from build123d import *

# Parameters (mm, degrees)
F0_R     = 53.0991394176
F1_DEPTH = 51.71754
F0_R_2   = 55.7255834594
F2_DEPTH = 232.41034
F3_T     = -2.54
F4_DEPTH = 228.21454
F5_T     = -2.54


# Not quite as in the source:
# - a shell that OpenCascade refuses in one call is made with other operations: the cavity is built on its own and cut out


with BuildPart() as f1:
    # F0 (on Top) → F1 (new body)
    with BuildSketch(Plane.XY):
        Circle(F0_R)
    extrude(amount=F1_DEPTH)

    # F3
    f3_openings = [f1.faces().sort_by_distance(p)[0] for p in [
        (0, 0, 51.71754),
    ]]
    offset(amount=F3_T, openings=f3_openings)

    # F4 (add): a face of the model
    f4_faces = [f1.faces().sort_by_distance(p)[0] for p in [
        (0, 0, 0),
    ]]


with BuildPart() as f2:
    # F0 (on Top) → F2 (new body)
    with BuildSketch(Plane.XY):
        Circle(F0_R_2)
        Circle(F0_R, mode=Mode.SUBTRACT)
    extrude(amount=-F2_DEPTH)


with BuildPart() as f1_1:
    add(f1.part)

    add(f2.part)  # F4 merges F2
    extrude(f4_faces, amount=F4_DEPTH)

    # F5: a shell. OpenCascade refuses it in one call, so the cavity is built on its own and cut out:
    # the body offset inwards by the wall thickness, plus a prism from it out through each open face.
    f5_core = offset(f1_1.part, amount=F5_T, kind=Kind.INTERSECTION, mode=Mode.PRIVATE)
    f5_exits = [f5_core.faces().sort_by_distance(p)[0] for p in [
        (0, 0, 0),
    ]]
    add(f5_core, mode=Mode.SUBTRACT)
    extrude(f5_exits, amount=-F5_T, mode=Mode.SUBTRACT)


solid = f1_1.part
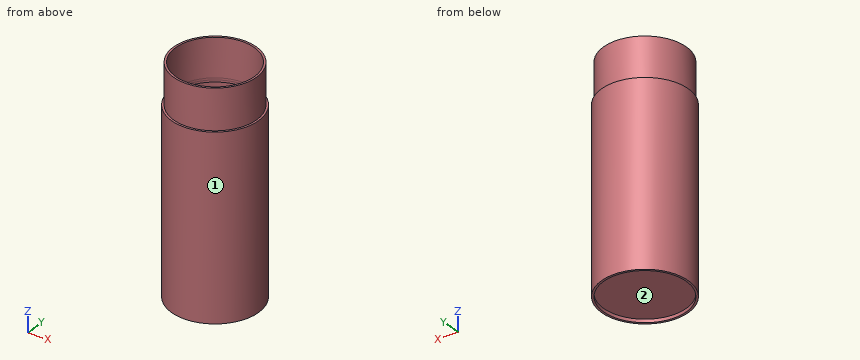
Source: CAD feature listing. Evaluate the final solid. Frame: model axes, mm. Face numbers are marked on the shaded views. Coordinates: 2 decimals unless noted, no trailing zeros. Order: outer loops, then holes, each group sorted by start corner. A loop starts at its lowest first (then second) coordinate and runs counter-clockwise, first axis right, second up. Notation, with made-up numbers: M 77.5,28.25 L 130.5,28.25 A21 cw 130.5,45.25 Z; hole C -2,60 d1. An arc over 180 degrees is marked long. Write each question's results on one line, items separated by ' | '. Start each with the question number.
1. Section D-D, the plane z = 21. Return the cut outline in (x, y).
2. Draft query along Y for the marked faces 1 and 2. Return one class per face: +Y half, -Y half, draft (parallel to the pull), parting line (faces both ways), or undercut.
3. Section C-C, the plane z = -89.5. Return the cut outline in (x, y), then the cut area to 3 significant figures.
4. Material intervals for L1, parallel to Z at x = 3, y = 51.5; L2, parallel to Y at x = 0, z = 33; L3, parallel to Y at x = 2, z = -15, sorted ascending.
5. Section A-A, the plane y = 0. Return the cut outline in (x, z).
6. Pin query (flat end, axial travel): pin 1 (1 mm diameter, centred on y = -41.5, z = -81.5, fed in from -X); pin 2 (3 mm diameter, centred on x = 18, z = 4.5, fed in from -Y); pin 3 (1 mm diameter, centred on x = 11.5, y = 6, fed in from +Z). Return the tip coordinate at first contact, or that it passes through.
Solution:
1) outline: C 0,0 d106.2; hole C 0,0 d101.12
2) face 1: parting line | face 2: undercut
3) outline: C 0,0 d111.45; hole C 0,0 d106.37 | area: 869 mm²
4) L1: -228.21 to -225.67, -2.54 to 51.72 | L2: -53.1 to -50.56, 50.56 to 53.1 | L3: -55.69 to -53.15, 53.15 to 55.69
5) outline: M -55.73,-232.41 L -53.1,-232.41 L -53.1,-228.21 L 53.1,-228.21 L 53.1,-232.41 L 55.73,-232.41 L 55.73,0 L 53.1,0 L 53.1,51.72 L 50.56,51.72 L 50.56,-2.54 L 53.19,-2.54 L 53.19,-225.67 L -53.19,-225.67 L -53.19,-2.54 L -50.56,-2.54 L -50.56,51.72 L -53.1,51.72 L -53.1,0 L -55.73,0 Z
6) pin 1: x = -37.74 | pin 2: y = -50.47 | pin 3: z = -225.67
